Job drawing, mm, ordinate dimensions from the low corner. One solid piece. A direction names the side the tool comes from. Give positions to 0.01 mm unless a question says otherwise; leave off trailing zeros. Write each loop counter-clockwise with the first axis right and the second up, starting at its lowest first coordinate (ties: lowest second). Pieces come first, ordered by that corner, then holes. Notation, with made-up numbers: M 80,52.5 L 111,52.5 A34 cw 111,87.5 Z; hole C -18,70.25 d5. An arc over 180 degrees is marked long. Use a Markdown table: item, result.
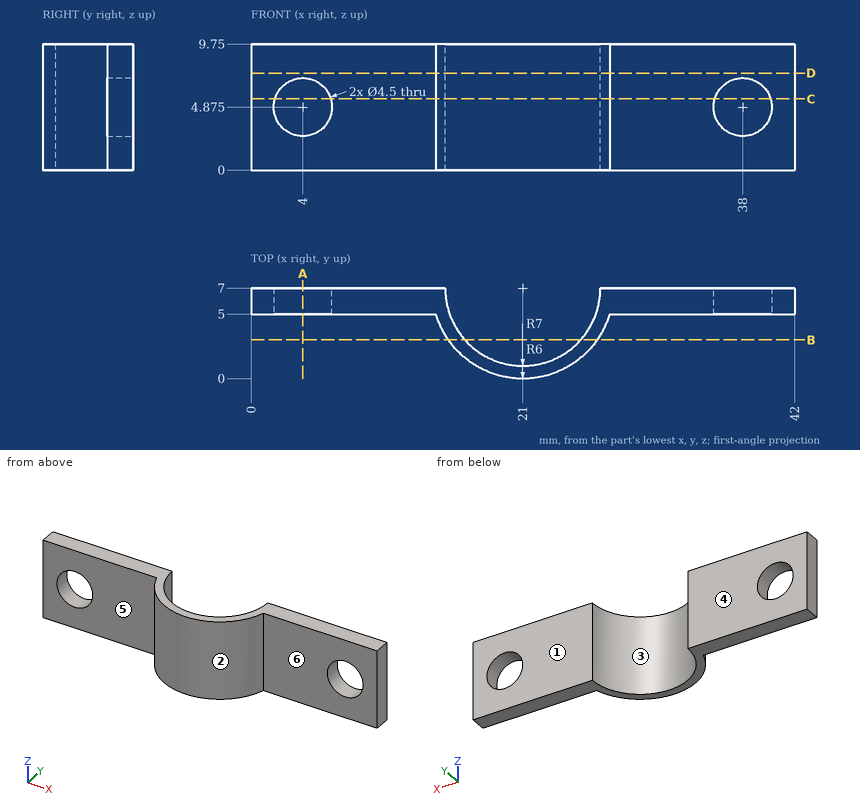
1. Drop flat-ended pins along their axis: P1, Ø3, axis at x = 35, z = 6, coming from the -Y side; P2, Ø3.5, axis at x = 38, z = 4.875, coming from the -Y side. Give the stop position or say it passes through.
Findings below:
| item | result |
|---|---|
| P1 | y = 5 |
| P2 | through |
2. Cut at B-B, the plane y = 3. Give the cut face in (x, z).
Findings below:
| item | result |
|---|---|
| outline | M 15.26,0 L 16.53,0 L 16.53,9.75 L 15.26,9.75 Z; M 25.47,0 L 26.74,0 L 26.74,9.75 L 25.47,9.75 Z |
3. Two-plate mould, pull along X, no slides. Class the marked faces 1, 2 and 3: released by +X, released by -X, zero draft, split by the parting line, or undercut.
Findings below:
| item | result |
|---|---|
| face 1 | zero draft |
| face 2 | split by the parting line |
| face 3 | undercut |
4. Cut at D-D, the plane z = 7.5. Give the cut face in (x, y), then the cut area to 3 significant figures.
Findings below:
| item | result |
|---|---|
| outline | M 0,5 L 14.29,5 A7 ccw 27.71,5 L 42,5 L 42,7 L 27,7 A6 cw 15,7 L 0,7 Z |
| area | 76.8 mm2 |
5. Tool access for the marked faces 4, 5 and 6: list every direction of +Z, -Z, +X, -X, +Y, -Y with a clear straight run to the whole face (end or side of a thin tool).
Findings below:
| item | result |
|---|---|
| face 4 | +Z, -Z, +X, -X, +Y |
| face 5 | +Z, -Z, -X, -Y |
| face 6 | +Z, -Z, +X, -Y |
6. Drill centre lines: L1, parallel to X at y = 6.75, z = 5.25; L2, parallel to Z at x = 4, y = 6.35 (3 decimals); L3, parallel to X at y = 5.5, z = 5.5. Where is each one in solid material? Low to high.
Findings below:
| item | result |
|---|---|
| L1 | 0 to 1.78, 6.22 to 15.01, 26.99 to 35.78, 40.22 to 42 |
| L2 | 0 to 2.625, 7.125 to 9.75 |
| L3 | 0 to 1.84, 6.16 to 15.19, 26.81 to 35.84, 40.16 to 42 |
7. Cut at C-C, the plane z = 5.5. Give the cut face in (x, y), then the cut area to 3 significant figures.
Findings below:
| item | result |
|---|---|
| outline | M 0,5 L 1.84,5 L 1.84,7 L 0,7 Z; M 6.16,5 L 14.29,5 A7 ccw 27.71,5 L 35.84,5 L 35.84,7 L 27,7 A6 cw 15,7 L 6.16,7 Z; M 40.16,5 L 42,5 L 42,7 L 40.16,7 Z |
| area | 59.5 mm2 |
8. Cut at A-A, the plane x = 4. Give the cut face in (y, z) (3 decimals).
Findings below:
| item | result |
|---|---|
| outline | M 5,0 L 7,0 L 7,2.625 L 5,2.625 Z; M 5,7.125 L 7,7.125 L 7,9.75 L 5,9.75 Z |
